Autodesk Inventor part; units mm, degrees
ref_plane "YZ Plane" through (0, 0, 0) normal (1, 0, 0) x (0, 1, 0)
ref_plane "XZ Plane" through (0, 0, 0) normal (0, 1, 0) x (-1, 0, 0)
ref_plane "XY Plane" through (0, 0, 0) normal (0, 0, 1) x (1, 0, 0)
sketch "Sketch2" plane through (0, 0, 0) normal (0, 0, 1) x (1, 0, 0)
  arc A0 (0, -57.15) -> (0, 57.15) centre (0, 0) ccw
  line L0 (241.3, 34.925) -> (241.3, -28.575)
  line L1 (-90.17, 0) -> (296.545, 0) construction
  arc A1 (0, -95.25) -> (26.7739, -91.4096) centre (0, 0) ccw
  arc A2 (24.2674, 92.1068) -> (0, 95.25) centre (0, 0) ccw
  line L2 (26.7739, -91.4096) -> (241.3, -28.575)
  line L3 (241.3, 34.925) -> (24.2674, 92.1068)
  line L4 (0, 95.25) -> (-12.7, 95.25)
  arc A3 (-12.7, 95.25) -> (-12.7, 57.15) centre (-12.7, 76.2) ccw
  line L5 (-12.7, 57.15) -> (0, 57.15)
  line L6 (0, -57.15) -> (-12.7, -57.15)
  arc A4 (-12.7, -57.15) -> (-12.7, -95.25) centre (-12.7, -76.2) ccw
  line L7 (-12.7, -95.25) -> (0, -95.25)
  circle A5 centre (-12.7, -76.2) radius 22.225 construction
  circle A6 centre (-12.7, 76.2) radius 22.225 construction
  line L8 (0, 137.795) -> (0, -137.795) construction
  point P0 (57.15, 0)
  point P1 (241.3, 3.175)
  dimension "d0" = 114.3
  dimension "d1" = 63.5
  dimension "d20" = 12.7
  dimension "d21" = 19.05
  dimension "d63" = 44.45
  dimension "d65" = 57.15
  dimension "d73" = 241.3
  dimension "d78" = 3.175
extrude "Plate1" add sketch "Sketch2" along normal blind 4.7625
sketch "Sketch3" plane through (0, 0, 4.7625) normal (0, 0, 1) x (1, 0, 0)
  line L0 (241.3, 34.925) -> (241.3, -28.575) construction
  line L1 (-86.36, 0) -> (295.91, 0) construction
  line L2 (228.6, 19.05) -> (228.6, -12.7) construction
  point P0 (0, 0)
  dimension "d7" = 31.75
  dimension "d8" = 12.7
  dimension "d75" = 19.05
hole "Hole1" at (228.6, 19.05, 4.7625) at (228.6, -12.7, 4.7625) direction (0, 0, -1) diameter 5.1054 end through all
pattern_linear "Rectangular Pattern1" count 5 spacing 25.4 along (-1, 0, 0) of "Hole1"
sketch "Sketch4" plane through (0, 0, 4.7625) normal (0, 0, 1) x (1, 0, 0)
  arc A0 (-12.7, 95.25) -> (-12.7, 57.15) centre (-12.7, 76.2) ccw construction
  arc A1 (-12.7, -57.15) -> (-12.7, -95.25) centre (-12.7, -76.2) ccw construction
  line L0 (-12.7, 76.2) -> (84.2314, 44.45) construction
  line L1 (-86.36, 0) -> (295.91, 0) construction
  line L2 (-12.7, -76.2) -> (84.2314, -44.45) construction
  circle A2 centre (84.2314, 44.45) radius 11.43 construction
  circle A3 centre (-12.7, 76.2) radius 11.43 construction
  line L3 (-9.1421, 87.0621) -> (87.7893, 55.3121) construction
  line L4 (-16.2579, 65.3379) -> (80.6735, 33.5879) construction
  line L5 (84.2314, 14.8167) -> (84.2314, -14.8167) construction
  point P0 (0, 0)
  point P1 (-12.7, -76.2)
  point P2 (84.2314, 0)
  dimension "d29" = 101.9988
  dimension "d30" = 44.45
  dimension "d38" = 22.86
  dimension "d39" = 29.6333
  dimension "d40" = 29.6333
  dimension "d41" = 29.6333
hole "Hole2" at (-12.7, 76.2, 4.7625) at (-12.7, -76.2, 4.7625) direction (0, 0, -1) diameter 28.575 end through all
hole "Hole3" at (84.2314, 44.45, 4.7625) at (84.2314, -44.45, 4.7625) at (84.2314, 14.8167, 4.7625) at (84.2314, -14.8167, 4.7625) direction (0, 0, -1) diameter 9.525 end through all
sketch "Sketch5" plane through (0, 0, 4.7625) normal (0, 0, 1) x (1, 0, 0)
  arc A0 (0, -57.15) -> (0, 57.15) centre (0, 0) ccw construction
  line L0 (-12.7, -57.15) -> (0, -57.15) construction
  arc A1 (-12.7, -57.15) -> (-12.7, -95.25) centre (-12.7, -76.2) ccw construction
  line L1 (0, -95.25) -> (-12.7, -95.25) construction
  arc A2 (0, -95.25) -> (26.7739, -91.4096) centre (0, 0) ccw construction
  line L2 (241.3, -28.575) -> (26.7739, -91.4096) construction
  line L3 (0, 57.15) -> (-12.7, 57.15) construction
  arc A3 (-12.7, 95.25) -> (-12.7, 57.15) centre (-12.7, 76.2) ccw construction
  line L4 (-12.7, 95.25) -> (0, 95.25) construction
  arc A4 (24.2674, 92.1068) -> (0, 95.25) centre (0, 0) ccw construction
  line L5 (24.2674, 92.1068) -> (241.3, 34.925) construction
  line L6 (197.4777, 33.3375) -> (105.4027, 57.5966)
  arc A5 (21.0318, 79.8259) -> (12.7, 81.5672) centre (0, 0) ccw
  arc A6 (69.85, 0) -> (53.5082, 44.8987) centre (0, 0) ccw construction
  line L7 (77.4255, 64.9677) -> (53.5082, 44.8987)
  line L8 (12.7, 81.5672) -> (12.7, 68.6858)
  line L9 (-86.36, 0) -> (295.91, 0) construction
  line L10 (241.3, 34.925) -> (241.3, -28.575) construction
  arc A7 (53.5082, 44.8987) -> (12.7, 68.6858) centre (0, 0) ccw
  line L11 (77.4255, 64.9677) -> (21.0318, 79.8259)
  line L12 (105.4027, 57.5966) -> (105.4027, 33.3375)
  line L13 (105.4027, 33.3375) -> (197.4777, 33.3375)
  line L14 (105.4027, 57.5966) -> (77.4255, 64.9677) construction
  line L15 (105.4027, -55.1457) -> (201.5387, -26.9875)
  line L16 (201.5387, -26.9875) -> (105.4027, -26.9875)
  line L17 (105.4027, -26.9875) -> (105.4027, -55.1457)
  circle A8 centre (152.4, 19.05) radius 2.5527 construction
  circle A9 centre (152.4, -12.7) radius 2.5527 construction
  point P0 (0, 0)
  dimension "d42" = 12.7
  dimension "d43" = 12.7
  dimension "d44" = 25.4
  dimension "d45" = 50
  dimension "d47" = 33.3375
  dimension "d48" = 92.075
  dimension "d66" = 12.7
  dimension "d67" = 26.9875
  dimension "d76" = 14.2875
  dimension "d77" = 14.2875
cut "Cut1" [suppressed]
cut "Cut2" [suppressed]
sketch "Sketch6" plane through (0, 0, 4.7625) normal (0, 0, 1) x (1, 0, 0)
  circle A0 centre (228.6, 19.05) radius 2.5527 construction
  circle A1 centre (203.2, -12.7) radius 2.5527 construction
  line L0 (228.6, 19.05) -> (203.2, -12.7) construction
  point P0 (0, 0)
  point P1 (215.9, 3.175)
hole "Hole4" at (215.9, 3.175, 4.7625) direction (0, 0, -1) diameter 22.225 end through all
pattern_linear "Rectangular Pattern2" count 5 spacing 25.4 along (-1, 0, 0) of "Hole4"
feature "Corner Round1" [suppressed]
mirror "Mirror2" [suppressed]
sketch "Sketch7" plane through (0, 0, 4.7625) normal (0, 0, 1) x (1, 0, 0)
  circle A0 centre (-12.7, 76.2) radius 14.2875 construction
  circle A1 centre (-12.7, -76.2) radius 14.2875 construction
  circle A2 centre (84.2314, -44.45) radius 4.7625 construction
  circle A3 centre (84.2314, 44.45) radius 4.7625 construction
  line L0 (84.2314, 44.45) -> (-12.7, 76.2) construction
  line L1 (-12.7, -76.2) -> (84.2314, -44.45) construction
  line L2 (59.9985, 52.3875) -> (64.9401, 67.4738) construction
  line L3 (59.9985, -52.3875) -> (64.9401, -67.4738) construction
  point P0 (0, 0)
  point P1 (35.7657, 60.325)
  point P2 (35.7657, -60.325)
  dimension "d86" = 25.4997
  dimension "d87" = 50.9994
  dimension "d88" = 25.4997
  dimension "d89" = 15.875
hole "Hole5" at (35.7657, 60.325, 4.7625) at (35.7657, -60.325, 4.7625) direction (0, 0, -1) diameter 6.35 end through all
fillet "Corner Round3" radius 6.35 2 edges at (241.3, -28.575, 2.3813) (241.3, 34.925, 2.3813)
equation "\"d14\" = Thickness"
equation "\"d66\" = d42"
equation "\"d49\" = Thickness"
equation "\"d68\" = Thickness"
equation "\"d84\" = Thickness"
equation "\"d6\" = Thickness"
equation "\"BendRadius\" = 1.5 * Thickness"
equation "\"BendReliefWidth\" = Thickness"
equation "\"BendReliefDepth\" = 0.5 * Thickness"
equation "\"CornerReliefSize\" = 4 * Thickness"
equation "\"MinimumRemnant\" = 2 * Thickness"
equation "\"TransitionRadius\" = BendRadius"
equation "\"JacobiRadiusSize\" = BendRadius"
equation "\"GapSize\" = Thickness"
properties part number "PLATE,END_EFFECTOR,ARM" material "Polycarbonate, Clear"
Here's how the part is built. I have some questions about the finished solid (model axes, mm). Give positions to 0.01 mm unless a question says otherwise; leave off trailing zeros. Write each loop counter-clockwise with the first axis right and the second up, starting at its lowest first coordinate (ties: lowest second). Pieces come first, ordered by that corner, then holes. Notation, with made-up numbers: (35.25, -8.5) -> (70.25, -8.5) arc R9 cw to (70.25, 7.5) -> close; hole circle Ø1 at (38, -7.75). An arc over 180 degrees is marked (long way). Use one line per item in the form item = value.
1) Suppose I cut it at B-B (y = 0). Please give me the cut outline in (x, z).
Verdict:
outline = (57.15, 0) -> (103.65, 0) -> (103.65, 4.76) -> (57.15, 4.76) -> close; (124.95, 0) -> (129.05, 0) -> (129.05, 4.76) -> (124.95, 4.76) -> close; (150.35, 0) -> (154.45, 0) -> (154.45, 4.76) -> (150.35, 4.76) -> close; (175.75, 0) -> (179.85, 0) -> (179.85, 4.76) -> (175.75, 4.76) -> close; (201.15, 0) -> (205.25, 0) -> (205.25, 4.76) -> (201.15, 4.76) -> close; (226.55, 0) -> (241.3, 0) -> (241.3, 4.76) -> (226.55, 4.76) -> close
2) Suppose I cut it at D-D (z = 2.7). Give the number of separate pieces and of enclosed holes in the cut face, and give its area (3 significant figures).
Verdict:
separate_pieces = 1
enclosed_holes = 23
area = 24,700 mm2
3) Suppose I cut it at A-A (x = 190.5). Please give me the cut outline in (y, z).
Verdict:
outline = (-43.45, 0) -> (-7.94, 0) -> (-7.94, 4.76) -> (-43.45, 4.76) -> close; (14.29, 0) -> (48.31, 0) -> (48.31, 4.76) -> (14.29, 4.76) -> close
4) We'd pull the mould along Y, two halves only. Please class faces 1 (the face through (103, 1, 4.762)), 2 (the face through (-13.328, 90.474, 2.348)), 3 (the face through (131.9, 63.75, 2.35)): +Y half, -Y half, draft (parallel to the pull), parting line (faces both ways), or undercut.
Verdict:
face_1 = draft
face_2 = undercut
face_3 = +Y half
5) If I drill on L1, parallel to Y at x = -13, z = 2.7; L2, parallel to Y at x = 83, z = 2.65; L3, parallel to X at y = -5.5, z = 0.2, over which ranges is the centre line in solid material (lowest first)? Write a range as [from, to].
Verdict:
L1 = [-95.25, -90.48], [-61.92, -57.15], [57.15, 61.92], [90.48, 95.25]
L2 = [-74.94, -49.05], [-39.85, -19.42], [-10.22, 10.22], [19.42, 39.85], [49.05, 76.63]
L3 = [56.88, 107.36], [121.24, 132.76], [146.64, 158.16], [172.04, 183.56], [197.44, 208.96], [222.84, 241.3]
6) Suppose I cut it at C-C (y = -72). Please give me the cut outline in (x, z), and give its area (3 significant figures).
Verdict:
outline = (-31.28, 0) -> (-26.36, 0) -> (-26.36, 4.76) -> (-31.28, 4.76) -> close; (0.96, 0) -> (93.04, 0) -> (93.04, 4.76) -> (0.96, 4.76) -> close
area = 462 mm2
7) I'm going to push flat-ended pins straight in: pin 1 (12.5 mm diameter, centred on x = 84.23, y = -44.45, fed in from -Z); pin 2 (2 mm diameter, centred on x = 118, z = 2.5, fed in from +Y). Where does each tip first touch, or does it pass through?
Verdict:
pin_1 = 0
pin_2 = 67.67
